Part print with two shaded views. Sizes in mm from the minimum x, y, z corner. Coordinates: 2 decimals unless noted, no trailing zeros. Order: outer loops, then holes, each group sorted by start corner. A loop starts at its lowest first (then second) coordinate and runs counter-clockwise, first axis right, second up. Notation, with made-up numbers: (-13.5, 71) - (32.5, 71) arc R12 ccw to (32.5, 89) - close; hole circle Ø6 at (26.25, -23.5). An arc over 180 degrees is marked (long way). Write each question's results on one line, items separated by ' | '. Start each with the question number.
Q1. Pin check, flat tips, straight feed: P1, Ø3, axis at y = 5, z = 16.5, coming from the +X side; P2, Ø2, axis at x = 59, y = 3, coming from the -Z side; P3, Ø2, axis at y = 3.5, z = 49, coming from the +X side; P4, Ø3, axis at y = 2.5, z = 32.5, coming from the -X side. Stop position of each tip, or through.
Q2. Wall check: probe 1 along Z at (x, y) = (64, 2.7); probe 2 along X at (y, z) = (1.55, 27.5); probe 3 along Z at (x, y) = (102.5, 5.1). Give the ranges that are in metal, low to high.
Q3. Band-saw the part on B-B, the plane y = 1.25. Write the cut outline in (x, z), then the cut area to 3 significant figures.
Q4. Band-saw the part on C-C, the plane z = 24. Write the cut outline in (x, y).
Q5. Band-saw the part on D-D, the plane x = 20. Write the cut outline in (y, z).
Q6. Band-saw the part on A-A, the plane x = 59. Write the cut outline in (y, z).
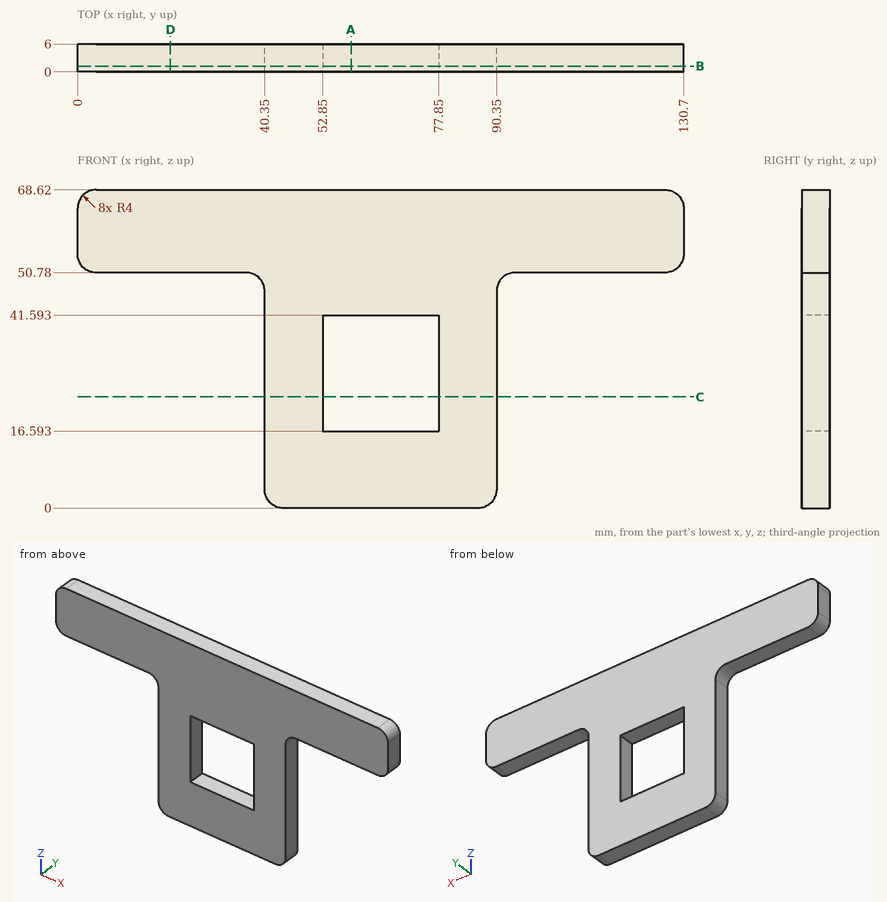
Results below:
1) P1: stops at x = 90.35 | P2: stops at z = 0 | P3: stops at x = 91.98 | P4: stops at x = 40.35
2) probe 1: z = 0 to 16.59, 41.59 to 68.62 | probe 2: x = 40.35 to 52.85, 77.85 to 90.35 | probe 3: z = 50.78 to 68.62
3) outline: (0, 54.78) arc R4 ccw to (4, 50.78) - (36.35, 50.78) arc R4 cw to (40.35, 46.78) - (40.35, 4) arc R4 ccw to (44.35, 0) - (86.35, 0) arc R4 ccw to (90.35, 4) - (90.35, 46.78) arc R4 cw to (94.35, 50.78) - (126.7, 50.78) arc R4 ccw to (130.7, 54.78) - (130.7, 64.62) arc R4 ccw to (126.7, 68.62) - (4, 68.62) arc R4 ccw to (0, 64.62) - close; hole (52.85, 16.59) - (77.85, 16.59) - (77.85, 41.59) - (52.85, 41.59) - close | area: 4,230 mm²
4) outline: (40.35, 0) - (52.85, 0) - (52.85, 6) - (40.35, 6) - close; (77.85, 0) - (90.35, 0) - (90.35, 6) - (77.85, 6) - close
5) outline: (0, 50.78) - (6, 50.78) - (6, 68.62) - (0, 68.62) - close
6) outline: (0, 0) - (6, 0) - (6, 16.59) - (0, 16.59) - close; (0, 41.59) - (6, 41.59) - (6, 68.62) - (0, 68.62) - close
